Here's how the part is built. I have some questions about the finished solid (model axes, mm). A direction names the side the tool comes from. Coordinates: 2 decimals unless noted, no trailing zeros. Write each loop counter-clockwise with the first axis right and the second up, starting at its lowest first coordinate (ties: lowest second). Pieces come first, ordered by that corner, then holes.
(1) Please list where these lines run through material, in increasing order: probe 1 along Z at (x, y) = (5.5, 3.1); probe 2 along X at (y, z) = (2.3, -111); probe 3 along Z at (x, y) = (-8, -9).
(2) Thinking about a two-plate mould opening in X: for faces 5 (the flat face through (0, 2, 14)), 6 (the flat face through (10, 2, -64)), 7 (the cylindrical face through (-5.87, 2.54, 11.16)), 8 (the flat face through (-0.8, -8, -91)), which applies, released by +X, released by -X, zero draft, split by the parting line, or undercut?
(3) Imagine slicing it at B-B, the plane x = 5.5. List the corners of the cut face in (y, z) for me, plus the area to 3 significant figures.
(4) Imagine slicing it at C-C, the plane y = -8. List the corners of the cut face in (x, z) for me.
(5) Which directions (+Z, -Z, +X, -X, +Y, -Y) give clear straight access to the entire face, cutting with the end or side of a thin tool? Please do faces 1 (the flat face through (5, -7, -14)), 2 (the flat face through (0.8, -8, -10)), 3 (the flat face through (0, 0, 10)), 4 (the flat face through (0, -15, -4)).
(6) Imagine slicing it at D-D, the plane z = -93.5. List the corners of the cut face in (x, y) for me.
(7) Imagine slicing it at A-A, the plane z = -111. List the corners of the cut face in (x, y) for me.
(8) For pin 1 Ø6.5 at (x, z) = (-2.5, 11.5) entering from -Y; pin 2 Ø1.8 at (x, y) = (0.5, -4.5) entering from +Z; pin 3 Ø3 at (x, y) = (-7.5, -8.5) entering from -Z, each with a flat end and sliding along its axis, tell me the tip position at first contact or that it passes through.
```python
from build123d import *

# Parameters (mm, degrees)
SKETCH1_W            = 20
SKETCH1_H            = 28
BOSS_EXTRUDE1_DEPTH  = 5
SKETCH2_W            = 20
SKETCH2_H            = 20
BOSS_EXTRUDE2_DEPTH  = 15
SKETCH3_W            = 1.6
SKETCH3_H            = 7.5
CUT_EXTRUDE1_DEPTH   = 15
M3_CLEARANCE_HOLE1_D = 3.4
SKETCH6_W            = 20
SKETCH6_H            = 5
BOSS_EXTRUDE3_DEPTH  = 93.5
SKETCH7_W            = 20
SKETCH7_H            = 5
BOSS_EXTRUDE4_DEPTH  = 8
SKETCH8_W            = 20
SKETCH8_H            = 20
BOSS_EXTRUDE5_DEPTH  = 15
SKETCH9_W            = 1.6
SKETCH9_H            = 35.5
CUT_EXTRUDE2_DEPTH   = 15
M3_CLEARANCE_HOLE2_D = 3.4


with BuildPart() as part:
    # Sketch1 → Boss-Extrude1 (new body)
    with BuildSketch(Plane(origin=(0, 0, 0), x_dir=(1, 0, 0), z_dir=(0, 1, 0))):
        Rectangle(SKETCH1_W, SKETCH1_H)
    extrude(amount=BOSS_EXTRUDE1_DEPTH)

    # Sketch2 → Boss-Extrude2 (add)
    with BuildSketch(Plane(origin=(0, 0, 0), x_dir=(-1, 0, 0), z_dir=(0, -1, 0))):
        with Locations((0, 4)):
            Rectangle(SKETCH2_W, SKETCH2_H)
    extrude(amount=BOSS_EXTRUDE2_DEPTH)

    # Sketch3 → Cut-Extrude1 (cut)
    with BuildSketch(Plane(origin=(0, -15, 0), x_dir=(-1, 0, 0), z_dir=(0, -1, 0))):
        with Locations((0, 10.25)):
            Rectangle(SKETCH3_W, SKETCH3_H)
    extrude(amount=-CUT_EXTRUDE1_DEPTH, mode=Mode.SUBTRACT)

    # M3 Clearance Hole1 (through all)
    with Locations(Plane(origin=(0, 0, 0), x_dir=(-1, 0, 0), z_dir=(0, -1, 0))):
        with Locations((-5.5, -9.5), (5.5, -9.5)):
            Hole(M3_CLEARANCE_HOLE1_D / 2)

    # Sketch6 → Boss-Extrude3 (add)
    with BuildSketch(Plane(origin=(0, 0, -14), x_dir=(-1, 0, 0), z_dir=(0, 0, -1))):
        with Locations((0, 2.5)):
            Rectangle(SKETCH6_W, SKETCH6_H)
    extrude(amount=BOSS_EXTRUDE3_DEPTH)

    # Sketch7 → Boss-Extrude4 (add)
    with BuildSketch(Plane(origin=(0, 0, -107.5), x_dir=(-1, 0, 0), z_dir=(0, 0, -1))):
        with Locations((0, 2.5)):
            Rectangle(SKETCH7_W, SKETCH7_H)
    extrude(amount=BOSS_EXTRUDE4_DEPTH)

    # Sketch8 → Boss-Extrude5 (add)
    with BuildSketch(Plane(origin=(0, 0, 0), x_dir=(-1, 0, 0), z_dir=(0, -1, 0))):
        with Locations((0, 97.5)):
            Rectangle(SKETCH8_W, SKETCH8_H)
    extrude(amount=BOSS_EXTRUDE5_DEPTH)

    # Sketch9 → Cut-Extrude2 (cut)
    with BuildSketch(Plane(origin=(0, -15, 0), x_dir=(-1, 0, 0), z_dir=(0, -1, 0))):
        with Locations((0, 77.75)):
            Rectangle(SKETCH9_W, SKETCH9_H)
    extrude(amount=-CUT_EXTRUDE2_DEPTH, mode=Mode.SUBTRACT)

    # M3 Clearance Hole2 (through all)
    with Locations(Plane(origin=(0, 0, 0), x_dir=(-1, 0, 0), z_dir=(0, -1, 0))):
        with Locations((-5.5, 111), (5.5, 111)):
            Hole(M3_CLEARANCE_HOLE2_D / 2)


solid = part.part
```
Recorded:
1. probe 1: z = -115.5 to -112.7, -109.3 to 7.8, 11.2 to 14
1. probe 2: x = -10 to -7.2, -3.8 to 3.8, 7.2 to 10
1. probe 3: z = -107.5 to -87.5, -14 to 6
2. face 5: zero draft
2. face 6: released by +X
2. face 7: undercut
2. face 8: undercut
3. outline: (-15, -107.5) - (0, -107.5) - (0, -109.3) - (5, -109.3) - (5, 7.8) - (0, 7.8) - (0, 6) - (-15, 6) - (-15, -14) - (0, -14) - (0, -87.5) - (-15, -87.5) - close; (0, -115.5) - (5, -115.5) - (5, -112.7) - (0, -112.7) - close; (0, 11.2) - (5, 11.2) - (5, 14) - (0, 14) - close
3. area: 1,210 mm2
4. outline: (-10, -107.5) - (10, -107.5) - (10, -87.5) - (0.8, -87.5) - (0.8, -95.5) - (-0.8, -95.5) - (-0.8, -87.5) - (-10, -87.5) - close; (-10, -14) - (-0.8, -14) - (-0.8, -6.5) - (0.8, -6.5) - (0.8, -14) - (10, -14) - (10, 6) - (-10, 6) - close
5. face 1: +X, -X, -Y
5. face 2: -Y
5. face 3: +Z, +X, -X, -Y
5. face 4: +Z, -Z, +X, -X, -Y
6. outline: (-10, -15) - (-0.8, -15) - (-0.8, 0) - (0.8, 0) - (0.8, -15) - (10, -15) - (10, 5) - (-10, 5) - close
7. outline: (-10, 0) - (-7.2, 0) - (-7.2, 5) - (-10, 5) - close; (-3.8, 0) - (3.8, 0) - (3.8, 5) - (-3.8, 5) - close; (7.2, 0) - (10, 0) - (10, 5) - (7.2, 5) - close
8. pin 1: stops at y = 0
8. pin 2: stops at z = 6
8. pin 3: stops at z = -107.5
